Here's how the part is built. I have some questions about the finished solid (model axes, mm). A direction names the side the tool comes from. Round coordinates to 2 decimals unless told otherwise and drop trailing zeros. Order: outer loops, then holes, each group sorted by start corner. A loop starts at its lowest first (then second) coordinate and runs counter-clockwise, first axis right, second up. Notation, with made-up numbers: M 84,-23.75 L 114,-23.75 A31 cw 114,6.25 Z; hole C 47.5,-31.5 d2. An arc over 180 degrees is marked long. Write item = value, one per line. Start each with the question number.
Item 1: I want a section at C-C, the plane z = -16. List the corners of the cut face in (x, y) for me.
Item 2: We'd pull the mould along X, two halves only. Please class faces 1 (the face through (64, 3, 8)), 2 (the face through (80.57, 3.45, -24.4)), 3 (the face through (74.46, 0.99, -5.59)): pulls with the +X half, pulls with the -X half, needs draft (parallel to the pull), parting line crosses it, or undercut.
Item 3: Please list where these lines run through material, in increasing order: L1, parallel to X at y = 5.1, z = -16; L2, parallel to Z at x = 70, y = 1.35; L3, parallel to X at y = 6.75, z = -5.
Item 4: For faces 4 (the face through (25, 4, 0)), 5 (the face through (25, 1, -10)), 6 (the face through (42, 7, -9)), 7 (the face through (5.912, 4.516, -15.005)), 8 (the face through (63.655, 4.028, -6.409)), which set-ups out of +Z, -Z, +X, -X, +Y, -Y let a thin tool reach every point of the face, with its end or its side?
Item 5: I want a section at D-D, the plane z = -4. List the corners of the cut face in (x, y) for me.
Item 6: I want a section at B-B, the plane y = 3.75. List the corners of the cut face in (x, z) for me, plus the area to 3 significant figures.
Item 7: I'm going to push flat-ended pins straight in: P1, Ø2, axis at x = 28, y = 3, coming from the +Z side; P2, Ø0.6, axis at y = 1.5, z = -5.5, coming from the -X side; P3, Ø3.5, axis at x = 5, z = -4, coming from the -Y side; P4, Ø7, axis at x = 70, z = -5, coming from the +Y side. Where does each tip first touch, or does it pass through?
Item 8: I want a section at A-A, the plane x = 5. List the corners of the cut face in (y, z) for me.
```python
from build123d import *

# Parameters (mm, degrees)
SKETCH1_R           = 4.5
BOSS_EXTRUDE1_DEPTH = 7
SKETCH2_W           = 25
SKETCH2_H           = 20
CUT_EXTRUDE1_DEPTH  = 2.1
SKETCH3_R           = 1.35
CUT_EXTRUDE2_DEPTH  = 14
FILLET2_R           = 3.5
SKETCH4_R           = 7.5
CUT_EXTRUDE3_DEPTH  = 1
SKETCH5_R           = 6.5
CUT_EXTRUDE4_DEPTH  = 4
FILLET3_R           = 15
SKETCH6_W           = 5
SKETCH6_H           = 5
BOSS_EXTRUDE2_DEPTH = 7
FILLET4_R           = 2


with BuildPart() as part:
    # Sketch1 → Boss-Extrude1 (new body)
    with BuildSketch(Plane(origin=(0, 0, 0), x_dir=(1, 0, 0), z_dir=(0, 1, 0))):
        Polygon((0, 0), (55, 0), (55, -8), (85, -8), (85, 0), (85, 20), (0, 20), align=None)
        with Locations(Location((70, 5, 0), (0, 0, 270))):
            Circle(SKETCH1_R, mode=Mode.SUBTRACT)
    extrude(amount=BOSS_EXTRUDE1_DEPTH)

    # Sketch2 → Cut-Extrude1 (cut)
    with BuildSketch(Plane.XZ):
        with Locations((12.5, -10)):
            Rectangle(SKETCH2_W, SKETCH2_H)
    extrude(amount=-CUT_EXTRUDE1_DEPTH, mode=Mode.SUBTRACT)

    # Sketch3 → Cut-Extrude2 (cut)
    with BuildSketch(Plane.XZ.offset(-2.1)):
        with Locations(Location((5, -4, 0), (0, 0, 270))):
            Circle(SKETCH3_R)
        with Locations(Location((20, -4, 0), (0, 0, 270))):
            Circle(SKETCH3_R)
        with Locations(Location((20, -16, 0), (0, 0, 270))):
            Circle(SKETCH3_R)
        with Locations(Location((5, -16, 0), (0, 0, 270))):
            Circle(SKETCH3_R)
    extrude(amount=-CUT_EXTRUDE2_DEPTH, mode=Mode.SUBTRACT)

    # Fillet2
    fillet2_edges = [part.edges().sort_by_distance(p)[0] for p in [
        (55, 3.5, 8),
        (55, 3.5, 0),
    ]]
    fillet(fillet2_edges, radius=FILLET2_R)

    # Sketch4 → Cut-Extrude3 (cut)
    with BuildSketch(Plane(origin=(0, 7, 0), x_dir=(1, 0, 0), z_dir=(0, 1, 0))):
        with Locations(Location((70, 5, 0), (0, 0, 270))):
            Circle(SKETCH4_R)
    extrude(amount=-CUT_EXTRUDE3_DEPTH, mode=Mode.SUBTRACT)

    # Sketch5 → Cut-Extrude4 (cut)
    with BuildSketch(Plane(origin=(0, 6, 0), x_dir=(1, 0, 0), z_dir=(0, 1, 0))):
        with Locations(Location((70, 5, 0), (0, 0, 270))):
            Circle(SKETCH5_R)
    extrude(amount=-CUT_EXTRUDE4_DEPTH, mode=Mode.SUBTRACT)

    # Fillet3
    fillet3_edges = [part.edges().sort_by_distance(p)[0] for p in [
        (85, 3.5, 8),
    ]]
    fillet(fillet3_edges, radius=FILLET3_R)

    # Sketch6 → Boss-Extrude2 (add)
    with BuildSketch(Plane(origin=(0, 7, 0), x_dir=(1, 0, 0), z_dir=(0, 1, 0))):
        with Locations((82.5, 22.5)):
            Rectangle(SKETCH6_W, SKETCH6_H)
    extrude(amount=-BOSS_EXTRUDE2_DEPTH)

    # Fillet4
    fillet4_edges = [part.edges().sort_by_distance(p)[0] for p in [
        (80, 3.5, -25),
        (80, 3.5, -20),
        (85, 3.5, -25),
    ]]
    fillet(fillet4_edges, radius=FILLET4_R)


solid = part.part
```
Filled in:
q1.outline = M 0,2.1 L 3.65,2.1 L 3.65,7 L 0,7 Z; M 6.35,2.1 L 18.65,2.1 L 18.65,7 L 6.35,7 Z; M 21.35,2.1 L 25,2.1 L 25,0 L 85,0 L 85,7 L 21.35,7 Z
q2.face_1 = needs draft
q2.face_2 = pulls with the -X half
q2.face_3 = undercut
q3.L1 = 0 to 3.65, 6.35 to 18.65, 21.35 to 85
q3.L2 = -20 to -9.5, -0.5 to 8
q3.L3 = 0 to 4.09, 5.91 to 19.09, 20.91 to 62.5, 77.5 to 84.87
q4.face_4 = +Z, -X, +Y, -Y
q4.face_5 = +Z, -Z, -X, -Y
q4.face_6 = +Z, -Z, +X, -X, +Y
q4.face_7 = +Y, -Y
q4.face_8 = +Y
q5.outline = M 0,2.1 L 3.65,2.1 L 3.65,7 L 0,7 Z; M 6.35,2.1 L 18.65,2.1 L 18.65,7 L 6.35,7 Z; M 21.35,2.1 L 25,2.1 L 25,0 L 65.61,0 L 65.61,2 L 63.58,2 L 63.58,6 L 62.57,6 L 62.57,7 L 21.35,7 Z; M 74.39,0 L 84.7,0 L 84.7,7 L 77.43,7 L 77.43,6 L 76.42,6 L 76.42,2 L 74.39,2 Z
q6.outline = M 0,-20 L 78,-20 A2 cw 80,-22 L 80,-23 A2 ccw 82,-25 L 83,-25 A2 ccw 85,-23 L 85,-7 A15 ccw 70,8 L 58.5,8 A3.5 ccw 55,4.5 L 55,3.5 A3.5 cw 51.5,0 L 0,0 Z; hole C 5,-16 d2.7; hole C 5,-4 d2.7; hole C 20,-16 d2.7; hole C 20,-4 d2.7; hole C 70,-5 d13
q6.area = 1,760 mm^2
q7.P1 = 0
q7.P2 = 25
q7.P3 = 2.1
q7.P4 = through
q8.outline = M 2.1,-20 L 7,-20 L 7,-17.35 L 2.1,-17.35 Z; M 2.1,-14.65 L 7,-14.65 L 7,-5.35 L 2.1,-5.35 Z; M 2.1,-2.65 L 7,-2.65 L 7,0 L 2.1,0 Z
